from build123d import *

# Parameters (mm, degrees)
SKETCH5_R           = 1.7859375
BOSS_EXTRUDE1_DEPTH = 1.5875
FILLET1_R           = 2.54


with BuildPart() as part:
    # Sketch5 → Boss-Extrude1 (new body)
    with BuildSketch(Plane.XY):
        with BuildLine():
            Line((89.745378764, 78.784933687), (88.224829537, 79.241098456))
            ThreePointArc((88.224829537, 79.241098456), (86.773324607, 79.32888397), (85.434920368, 78.760335862))
            Line((85.434920368, 78.760335862), (79.568453922, 74.458260468))
            ThreePointArc((79.568453922, 74.458260468), (83.306311174, 69.347675041), (89.593323842, 68.597253861))
            Line((89.593323842, 68.597253861), (109.072532015, 69.929775894))
            Line((109.072532015, 69.929775894), (133.35, 65.0875))
            Line((133.35, 65.0875), (140.381467098, 62.743677634))
            Line((140.381467098, 62.743677634), (145.272774991, 77.417601312))
            Line((145.272774991, 77.417601312), (137.366092628, 80.0531621))
            Line((137.366092628, 80.0531621), (135.860057893, 75.535057893))
            Line((135.860057893, 75.535057893), (134.354023157, 76.037069471))
            ThreePointArc((134.354023157, 76.037069471), (133.228154551, 76.197661136), (132.117919025, 75.951192316))
            Line((132.117919025, 75.951192316), (125.413170132, 73.128140151))
            Line((125.413170132, 73.128140151), (122.383992203, 80.322437731))
            Line((122.383992203, 80.322437731), (112.493298596, 84.486940303))
            Line((112.493298596, 84.486940303), (110.645177133, 80.097651828))
            Line((110.645177133, 80.097651828), (109.182080975, 80.713692316))
            ThreePointArc((109.182080975, 80.713692316), (107.712055506, 80.953571291), (106.29439622, 80.496669822))
            Line((106.29439622, 80.496669822), (100.08690833, 76.703205))
            Line((100.08690833, 76.703205), (97.130029166, 81.541734542))
            Line((97.130029166, 81.541734542), (91.113873069, 83.346581371))
            Line((91.113873069, 83.346581371), (89.745378764, 78.784933687))
        make_face()
        with Locations((140.880173678, 75.535057893)):
            Circle(SKETCH5_R, mode=Mode.SUBTRACT)
        with Locations((115.650506095, 79.712626524)):
            Circle(SKETCH5_R, mode=Mode.SUBTRACT)
        with Locations((94.763191216, 78.93698861)):
            Circle(SKETCH5_R, mode=Mode.SUBTRACT)
    extrude(amount=BOSS_EXTRUDE1_DEPTH)

    # Fillet1
    fillet1_edges = [part.edges().sort_by_distance(p)[0] for p in [
        (109.072532015, 69.929775894, 0.79375),
        (79.568453922, 74.458260468, 0.79375),
        (91.113873069, 83.346581371, 0.79375),
        (97.130029166, 81.541734542, 0.79375),
        (112.493298596, 84.486940303, 0.79375),
        (122.383992203, 80.322437731, 0.79375),
        (137.366092628, 80.0531621, 0.79375),
        (145.272774991, 77.417601312, 0.79375),
        (140.381467098, 62.743677634, 0.79375),
        (133.35, 65.0875, 0.79375),
    ]]
    fillet(fillet1_edges, radius=FILLET1_R)


solid = part.part
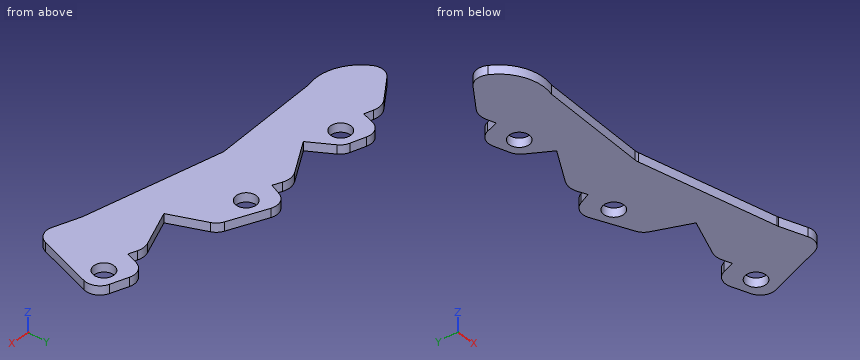
Geometry: final body of the model. Coordinates: model frame, mm. Round coordinates to 2 decimals unless told otherwise and drop trailing zeros. Loops run counter-clockwise (first coordinate to the right, second up) from the corner with the lowest first, then second, coordinate; pieces in that order, holes last.
Q1. Section D-D on x = 98.5. Return loops of the section in (y, z), plus the area to 3 significant figures.
Q2. Section B-B on x = 130. Return loops of the section in (y, z), plus the area to 3 significant figures.
Q3. Pin query (flat end, axial travel): P1, Ø8, axis at x = 130.5, y = 80, coming from the +Z side. Return the tip coordinate at first contact, or that it passes through.
Q4. Section C-C on z = 0.75. State how many separate pieces and enclosed holes the cut face has, plus the area to 3 significant figures.
Q5. Material intervals for L1, parallel to Y at x = 139, z = 1.1; L2, parallel to Y at x = 140, z = 0.65; L3, parallel to Y at x = 90.5, z = 0.45, sorted ascending.
Q6. Section A-A on y = 69.25. Return loops of the section in (x, z).
Evaluation:
1. outline: (69.21, 0) - (79.3, 0) - (79.3, 1.59) - (69.21, 1.59) - close
1. area: 16.0 mm2
2. outline: (65.76, 0) - (75.06, 0) - (75.06, 1.59) - (65.76, 1.59) - close
2. area: 14.8 mm2
3. P1: passes through
4. separate pieces: 1
4. enclosed holes: 3
4. area: 679 mm2
5. L1: y = 63.43 to 79.38
5. L2: y = 63.73 to 73.98, 77.09 to 79.18
5. L3: y = 68.66 to 81.22
6. outline: (83.48, 0) - (99.14, 0) - (99.14, 1.59) - (83.48, 1.59) - close; (112.48, 0) - (142.55, 0) - (142.55, 1.59) - (112.48, 1.59) - close
